```python
from build123d import *

# Parameters (mm, degrees)
F1_DEPTH = 177.8
F3_DEPTH = 172.466


# Not quite as in the source:
# - a feature names something its author has since deleted; it is built from what else it names


with BuildPart() as f1:
    # F0 (on Front) → F1 (new body)
    with BuildSketch(Plane.XZ):
        with BuildLine():
            ThreePointArc((-32.1100279689, 0), (-22.7052185209, 22.7052185209), (0, 32.1100279689))
            ThreePointArc((0, 32.1100279689), (22.7052185209, 22.7052185209), (32.1100279689, 0))
            Line((32.1100279689, 0), (38.3662581444, 0))
            ThreePointArc((38.3662581444, 0), (27.1290413026, 27.1290413026), (0, 38.3662581444))
            ThreePointArc((0, 38.3662581444), (-27.1290413026, 27.1290413026), (-38.3662581444, 0))
            Line((-38.3662581444, 0), (-32.1100279689, 0))
        make_face()
    extrude(amount=F1_DEPTH)

    # F2 (on face) → F3 (join)
    with BuildSketch(Plane.XZ.offset(177.8)):
        Polygon((-26.2182112783, 38.40040043), (-9.5876645925, 0), (0, 0), (8.5017651877, 0), (25.3681559116, 37.5649854541), (20.6263340544, 40.6422178311), (5.2554043941, 5.8927594628), (-5.9924047246, 5.8927594628), (-21.0417917943, 40.6422178311), align=None)
    extrude(amount=-F3_DEPTH)


solid = f1.part
```
Source: CAD feature listing. Evaluate the final solid. Frame: model axes, mm. A direction names the side the tool comes from. Give positions to 0.01 mm unless a question says otherwise; leave off trailing zeros. Order: outer loops, then holes, each group sorted by start corner. A loop starts at its lowest first (then second) coordinate and runs counter-clockwise, first axis right, second up.
(1) Contact query for flat-ended pins moving along their axis: P1, Ø6, axis at x = -19, y = -111.5, coming from the +Z side; P2, Ø12, axis at x = -18.5, z = 4, coming from the +Y side; P3, Ø12, axis at y = -140.5, z = 9.5, coming from the -X side; P4, Ø2, axis at y = -123.5, z = 13, coming from the +X side. Output: stop coordinate, or through.
(2) Material intervals for line 1 along X through (y, z) = (-57.5, 14); line 2 along X through (y, z) = (-148, 7.5); line 3 along X through (y, z) = (-147, 3), sorted ascending.
(3) Section query A-A (y = -35.5). Return the cut outline in (x, z).
(4) Section query B-B (z = 11). Return the cut outline in (x, y), plus the area to 3 significant figures.
(5) Access query for faces 1 (the face through (19.186, -92.774, 37.386)), 2 (the face through (14.09, -92.77, 12.45)), 3 (the face through (-24.59, -92.77, 34.64)), 4 (the face through (-3, -5.334, 5)), 5 (the face through (0, -93, 5.893)). Directions: +Z, -Z, +X, -X, +Y, -Y. A direction counts if a zero-diameter tool reaches every point of the face in a straight line with its end or side. Return the directions, or none.
(6) Pull-direction query (Z, two-part tool) for faces 6 (the face through (23, -92.8, 39.1)), 7 (the face through (-10.73, -92.77, 16.83)), 8 (the face through (23.897, -92.774, 34.288)), 9 (the face through (-1, -93, 0)); classes: +Z half, -Z half, draft (parallel to the pull), parting line (faces both ways), or undercut.
Outcome:
1. P1: stops at z = 40.64
1. P2: passes through
1. P3: stops at x = -38.21
1. P4: stops at x = 36.44
2. line 1: x = -35.72 to -28.9, -15.65 to -9.5, 8.84 to 14.79, 28.9 to 35.72
2. line 2: x = -37.63 to -31.22, -12.84 to -6.69, 5.97 to 11.87, 31.22 to 37.63
2. line 3: x = -38.25 to -31.97, -10.89 to 9.85, 31.97 to 38.25
3. outline: (-38.37, 0) - (-32.11, 0) arc R32.11 cw to (-20.35, 24.84) - (-9.59, 0) - (8.5, 0) - (19.84, 25.25) arc R32.11 cw to (32.11, 0) - (38.37, 0) arc R38.37 ccw to (22.47, 31.1) - (25.37, 37.56) - (20.63, 40.64) - (17.7, 34.04) arc R38.37 ccw to (-18.09, 33.83) - (-21.04, 40.64) - (-26.22, 38.4) - (-22.91, 30.77) arc R38.37 ccw to start; hole (-15.6, 28.07) - (-5.99, 5.89) - (5.26, 5.89) - (15.17, 28.3) arc R32.11 ccw to start
4. outline: (-36.76, -177.8) - (-30.17, -177.8) - (-30.17, 0) - (-36.76, 0) - close; (-14.35, -177.8) - (-8.2, -177.8) - (-8.2, -5.33) - (-14.35, -5.33) - close; (7.51, -177.8) - (13.44, -177.8) - (13.44, -5.33) - (7.51, -5.33) - close; (30.17, -177.8) - (36.76, -177.8) - (36.76, 0) - (30.17, 0) - close
4. area: 4,430 mm2
5. face 1: +Z, +Y, -Y
5. face 2: -Z, +Y, -Y
5. face 3: -X, +Y, -Y
5. face 4: -Z, +Y
5. face 5: +Y, -Y
6. face 6: +Z half
6. face 7: undercut
6. face 8: undercut
6. face 9: -Z half
